Verification items for the finished model (mm, model axes). Face numbers are marked on the shaded views. A direction names the side the tool comes from. Give positions to 0.01 mm unless a question says otherwise; leave off trailing zeros. Order: outer loops, then holes, each group sorted by start corner. A loop starts at its lowest first (then second) coordinate and runs counter-clockwise, first axis right, second up. Notation, with made-up numbers: (6, -33.75) -> (18, -33.75) arc R20 cw to (18, -4.75) -> close; hole circle Ø4 at (7.25, 59.5). An arc over 180 degrees is marked (long way). One line per question, with ' | ' between items. Start each with the question number.
Q1. Section check A-A on y = -8.5. Record the cut outline in (x, z) (3 decimals).
Q2. Access from +Z, -Z, +X, -X, +Y, -Y to the whole of each face (thin tool, end or side, straight path). Record for the marked faces 1, 2 and 3.
Q3. Go/stop test with a flat-tipped pin: pin 1 (0.5 mm diameter, centred on x = 2.5, z = 0, fed in from -Y). Record where the tip stops, or that it passes through.
Q4. Material ranges on probe 1 along X at (y, z) = (-1, 0) (3 decimals); probe 2 along Z at (x, y) = (0, -16.5) (3 decimals); probe 3 along X at (y, z) = (19, -0.45), recorded low to high. Write a range as [from, to].
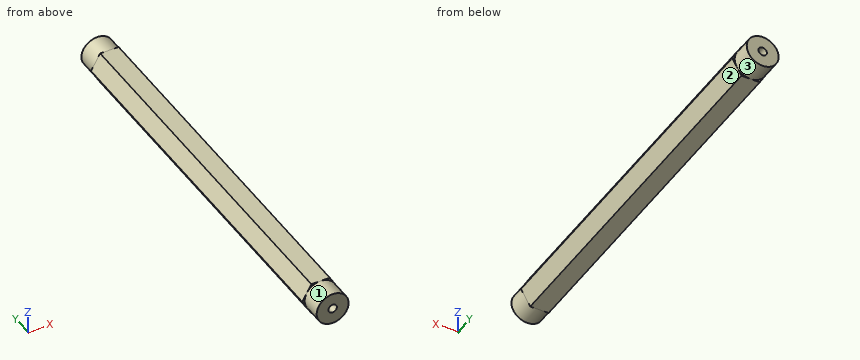
from build123d import *

# Parameters (mm, degrees)
SKETCH1_R           = 0.635
BOSS_EXTRUDE1_DEPTH = 27.813
SKETCH2_R           = 2.38125
SKETCH2_R_2         = 0.635
BOSS_EXTRUDE2_DEPTH = 3.175
SKETCH3_R           = 2.38125
SKETCH3_R_2         = 0.635
BOSS_EXTRUDE3_DEPTH = 3.175


with BuildPart() as part:
    # Sketch1 → Boss-Extrude1 (new body, symmetric)
    with BuildSketch(Plane(origin=(0, 0, 0), x_dir=(1, 0, 0), z_dir=(0, 1, 0))):
        Polygon((1.374815329, -2.38125), (2.749630657, 0), (1.374815329, 2.38125), (-1.374815329, 2.38125), (-2.749630657, 0), (-1.374815329, -2.38125), align=None)
        Circle(SKETCH1_R, mode=Mode.SUBTRACT)
    extrude(amount=BOSS_EXTRUDE1_DEPTH, both=True)

    # Sketch2 → Boss-Extrude2 (add)
    with BuildSketch(Plane(origin=(0, 27.813, 0), x_dir=(1, 0, 0), z_dir=(0, 1, 0))):
        Circle(SKETCH2_R)
        Circle(SKETCH2_R_2, mode=Mode.SUBTRACT)
    extrude(amount=BOSS_EXTRUDE2_DEPTH)

    # Sketch3 → Boss-Extrude3 (add)
    with BuildSketch(Plane.XZ.offset(27.813)):
        Circle(SKETCH3_R)
        Circle(SKETCH3_R_2, mode=Mode.SUBTRACT)
    extrude(amount=BOSS_EXTRUDE3_DEPTH)


solid = part.part
Filled in:
1) outline: (-2.75, 0) -> (-1.375, -2.381) -> (1.375, -2.381) -> (2.75, 0) -> (1.375, 2.381) -> (-1.375, 2.381) -> close; hole circle Ø1.27 at (0, 0)
2) face 1: -Y | face 2: -Z, +X, +Y, -Y | face 3: +Y
3) pin 1: y = -30.99
4) probe 1: [-2.75, -0.635], [0.635, 2.75] | probe 2: [-2.381, -0.635], [0.635, 2.381] | probe 3: [-2.49, -0.45], [0.45, 2.49]
